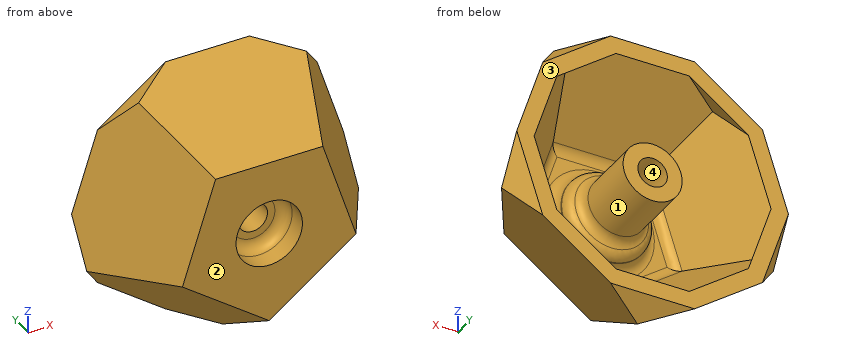
from build123d import *

# Parameters (mm, degrees)
BOSS_EXTRUDE1_DEPTH     = 30
BOSS_EXTRUDE1_TAPER     = -26.56505118
SKETCH3_OUTSIDE_W       = 108.076
SKETCH3_OUTSIDE_H       = 105.2
CUT_EXTRUDE1_DEPTH      = 30
CUT_EXTRUDE1_TAPER      = 26.56505118
SKETCH5_R               = 19.347524159
CUT_EXTRUDE2_DEPTH      = 25
SHELL1_T                = -2
SKETCH6_R               = 4
SKETCH6_R_2             = 2
BOSS_EXTRUDE2_DEPTH     = 13
SKETCH10_R              = 6
SKETCH10_R_2            = 4
BOSS_EXTRUDE4_DEPTH     = 3
FILLET5_R               = 1.5
SKETCH10_3_R            = 4.5
SKETCH10_3_R_2          = 4
CUT_EXTRUDE3_DEPTH      = 2
CUT_EXTRUDE3_DEPTH_BACK = 2
FILLET6_R               = 1.5


with BuildPart() as part:
    # Sketch1 → Boss-Extrude1 (new body)
    with BuildSketch(Plane(origin=(0, 0, 0), x_dir=(1, 0, 0), z_dir=(0, 1, 0))):
        Polygon((0, 12.360679775), (-11.755705046, 3.819660113), (-7.26542528, -10), (7.26542528, -10), (11.755705046, 3.819660113), align=None)
    extrude(amount=BOSS_EXTRUDE1_DEPTH, taper=BOSS_EXTRUDE1_TAPER)

    # Sketch3 outside → Cut-Extrude1 (cut)
    with BuildSketch(Plane(origin=(0, 30, 0), x_dir=(1, 0, 0), z_dir=(0, 1, 0))):
        with Locations((0, 2.951)):
            Rectangle(SKETCH3_OUTSIDE_W, SKETCH3_OUTSIDE_H)
        Polygon((7.26542528, 10), (-7.26542528, 10), (-11.755705046, -3.819660113), (0, -12.360679775), (11.755705046, -3.819660113), align=None, mode=Mode.SUBTRACT)
    extrude(amount=-CUT_EXTRUDE1_DEPTH, taper=CUT_EXTRUDE1_TAPER, mode=Mode.SUBTRACT)

    # Sketch5 → Cut-Extrude2 (cut)
    with BuildSketch(Plane(origin=(0, 15, 0), x_dir=(1, 0, 0), z_dir=(0, 1, 0))):
        Circle(SKETCH5_R)
    extrude(amount=CUT_EXTRUDE2_DEPTH, mode=Mode.SUBTRACT)

    # Shell1
    shell1_openings = [part.faces().sort_by_distance(p)[0] for p in [
        (0, 15, 0),
    ]]
    offset(amount=SHELL1_T, openings=shell1_openings, kind=Kind.INTERSECTION)

    # Sketch6 → Boss-Extrude2 (add)
    with BuildSketch(Plane(origin=(0, 2, 0), x_dir=(1, 0, 0), z_dir=(0, 1, 0))):
        with Locations(Location((0, 0, 0), (0, 0, 270))):
            Circle(SKETCH6_R)
        with Locations(Location((0, 0, 0), (0, 0, 270))):
            Circle(SKETCH6_R_2, mode=Mode.SUBTRACT)
    extrude(amount=BOSS_EXTRUDE2_DEPTH)

    # Sketch10 → Boss-Extrude4 (add)
    with BuildSketch(Plane(origin=(0, 2, 0), x_dir=(1, 0, 0), z_dir=(0, 1, 0))):
        with Locations(Location((0, 0, 0), (0, 0, 270))):
            Circle(SKETCH10_R)
        with Locations(Location((0, 0, 0), (0, 0, 270))):
            Circle(SKETCH10_R_2, mode=Mode.SUBTRACT)
    extrude(amount=BOSS_EXTRUDE4_DEPTH)

    # Fillet5
    fillet5_edges = [part.edges().sort_by_distance(p)[0] for p in [
        (0, 2, -6),
        (0, 5, -4),
        (5.151309995, 2, -7.090169944),
        (-5.151309995, 2, -7.090169944),
        (-8.334994658, 2, 2.708203933),
        (0, 2, 8.763932023),
        (8.334994658, 2, 2.708203933),
    ]]
    fillet(fillet5_edges, radius=FILLET5_R)

    # Sketch10<3> → Cut-Extrude3 (cut, two sides)
    with BuildSketch(Plane(origin=(0, 2, 0), x_dir=(1, 0, 0), z_dir=(0, 1, 0))) as cut_extrude3_sk:
        with Locations(Location((0, 0, 0), (0, 0, 270))):
            Circle(SKETCH10_3_R)
        with Locations(Location((0, 0, 0), (0, 0, 270))):
            Circle(SKETCH10_3_R_2, mode=Mode.SUBTRACT)
        with Locations(Location((0, 0, 0), (0, 0, 270))):
            Circle(SKETCH10_3_R_2)
    extrude(amount=CUT_EXTRUDE3_DEPTH, mode=Mode.SUBTRACT)
    extrude(cut_extrude3_sk.sketch, amount=-CUT_EXTRUDE3_DEPTH_BACK, mode=Mode.SUBTRACT)

    # Fillet6
    fillet6_edges = [part.edges().sort_by_distance(p)[0] for p in [
        (0, 4, -4.5),
        (0, 5, -6),
    ]]
    fillet(fillet6_edges, radius=FILLET6_R)


solid = part.part
Source: CAD feature listing. Evaluate the final solid. Frame: model axes, mm. Face numbers are marked on the shaded views. A direction names the side the tool comes from. Round coordinates to 2 decimals unless told otherwise and drop trailing zeros. Answer as a JSON object with one key per item and string values. Group by question number.
Q1. Section query A-A (y = 13). State how many separate pieces and enclosed holes the cut face has, plus the area to 3 significant figures.
Q2. Ray query, line 1 (Z direction, x = -2.5, y = 12); line 2 (X direction, y = 7.75, z = -1); line 3 (X direction, y = 1.75, z = 0). Return the intervals inside material, ascending. Write a range as from..to.
Q3. Access query for the marked faces 1 and 2. Directions: +Z, -Z, +X, -X, +Y, -Y. A direction counts if a zero-diameter tool reaches every point of the face in a straight line with its end or side. Return the directions, or none.
Q4. Mould query, pull axis X, two halves, no side actions, for the marked faces 3 and 4. Classes: pulls with the +X half, pulls with the -X half, needs draft (parallel to the pull), parting line crosses it, or undercut.
Q5. Contact query for flat-ended pins moving along their axis: P1, Ø1.5, axis at x = 2.5, z = -8, coming from the +Y side; P2, Ø3, axis at y = 7, z = -9.5, coming from the +X side; P3, Ø5, axis at y = 12.5, z = -7.5, coming from the +X side; P4, Ø3, axis at x = 0, z = 0, coming from the +Y side. Output: stop coordinate, or through.
Completed:
{
 "1": {"separate pieces": "2", "enclosed holes": "2", "area": "276 mm²"},
 "2": {"line 1": "-17.96..-15.2, -3.12..3.12, 13.76..16", "line 2": "-14.91..-12.56, -3.87..-1.73, 1.73..3.87, 12.56..14.91", "line 3": "-11.43..-4.5, 4.5..11.43"},
 "3": {"face 1": "+Y", "face 2": "+Z, -Z, +X, -X, -Y"},
 "4": {"face 3": "needs draft", "face 4": "undercut"},
 "5": {"P1": "y = 2.27", "P2": "x = 12.32", "P3": "x = 18.4", "P4": "through"}
}
